Work out the finished part from the listing and answer in its coordinate system (mm). Round coordinates to 2 decimals unless told otherwise and drop trailing zeros. Write each loop counter-clockwise with the first axis right and the second up, starting at its lowest first coordinate (ties: lowest second). Pieces come first, ordered by that corner, then holes. Notation, with made-up numbers: M -4,-10.75 L 36,-10.75 A18 cw 36,-3.75 Z; hole C 29.25,73.5 d4. An arc over 180 degrees is marked long. Answer in a Markdown table with one row per item.
Autodesk Inventor part; units mm, degrees
ref_plane "YZ Plane" through (0, 0, 0) normal (1, 0, 0) x (0, 1, 0)
ref_plane "XZ Plane" through (0, 0, 0) normal (0, 1, 0) x (-1, 0, 0)
ref_plane "XY Plane" through (0, 0, 0) normal (0, 0, 1) x (1, 0, 0)
sketch "Sketch1" plane through (0, 0, 0) normal (0, 1, 0) x (-1, 0, 0)
  line L0 (0, 0) -> (48.3, 0)
  line L1 (48.3, 0) -> (48.3, -15)
  line L2 (48.3, -15) -> (0, -15)
  line L3 (0, -15) -> (0, 0)
  circle A0 centre (48.3, 0) radius 1.5
  circle A1 centre (48.3, -15) radius 1.5
  circle A2 centre (0, 0) radius 1.5
  circle A3 centre (0, -15) radius 1.5
  line L4 (48.3, -15) -> (52.3, -15)
  line L5 (52.3, -15) -> (52.3, -17.5)
  line L6 (52.3, -17.5) -> (48.3, -17.5)
  line L7 (48.3, -17.5) -> (48.3, -15)
  line L8 (0, 0) -> (-4, 0)
  line L9 (-4, 0) -> (-4, 2.5)
  line L10 (-4, 2.5) -> (0, 2.5)
  line L11 (0, 2.5) -> (0, 0)
  line L12 (-4, 2.5) -> (52.3, 2.5)
  line L13 (52.3, 2.5) -> (52.3, -17.5)
  line L14 (52.3, -17.5) -> (-4, -17.5)
  line L15 (-4, -17.5) -> (-4, 2.5)
  dimension "d0" = 48.3
  dimension "d1" = 15
  dimension "d2" = 3
  dimension "d3" = 3
  dimension "d4" = 3
  dimension "d5" = 3
  dimension "d6" = 4
  dimension "d7" = 2.5
  dimension "d8" = 4
  dimension "d9" = 2.5
extrude "Extrusion1" add sketch "Sketch1" along normal blind 2 contours A2 L11 L12 L13 L4 A1 L1 A0 L0 | L0 A0 L1 A1 L2 A3 L3 A2 | L3 A3 L2 A1 L7 L14 L15 L8 A2 | L8 L9 L10 L11 A2 | L7 A1 L4 L5 L6
sketch "Sketch2" plane through (0, 2, 0) normal (0, 1, 0) x (1, 0, 0)
  line L0 (4, -2.5) -> (4, 17.5)
  line L1 (4, -2.5) -> (-14.15, -2.5)
  line L2 (-14.15, -2.5) -> (-14.15, 7.5)
  line L3 (-14.15, 7.5) -> (4, 7.5)
  line L4 (4, 7.5) -> (4, -2.5)
  circle A0 centre (-14.15, 7.5) radius 3
  circle A1 centre (-14.15, 7.5) radius 1.5
  point P0 (0, 0)
  dimension "d12" = 18.15
  dimension "d13" = 10
  dimension "d14" = 6
  dimension "d19" = 3
extrude "Extrusion2" add sketch "Sketch2" along normal blind 1 contours A0 L2 A1 L3 | L3 A1 L2 A0
extrude "Extrusion3" cut sketch "Sketch2" against normal blind 3 contours A1 L2 L3 | L3 L2 A1
fillet "Fillet2" radius 2 1 edges at (-17.15, 2, -7.5)
properties part number "back_servo_support"
1. Determine the mould class of faces 1 (the flat face through (-24, 2, -7)), 2 (the cylindrical face through (-49.73, 0.99, -15.45)), 3 (the cylindrical face through (1.5, 0.99, -0.07)), 4 (the flat face through (-52.3, 1, -7)) for opening direction X: released by +X, released by -X, zero draft, split by the parting line, or undercut.
Calculated:
| item | result |
|---|---|
| face 1 | zero draft |
| face 2 | undercut |
| face 3 | undercut |
| face 4 | released by -X |
2. The part is cut by section A-A (x = 0). Determine the outline of the cut face in (y, z).
Calculated:
| item | result |
|---|---|
| outline | M 0,-17.5 L 2,-17.5 L 2,-16.5 L 0,-16.5 Z; M 0,-13.5 L 2,-13.5 L 2,-1.5 L 0,-1.5 Z; M 0,1.5 L 2,1.5 L 2,2.5 L 0,2.5 Z |
3. Consider line 1 along Z through (x, y) = (-48.3, 1); line 2 along X through (y, z) = (1.25, 0); line 3 along Z through (x, y) = (-47.5, 1.45). Determine where each line is inside the solid, lowest interval first. Write a range as from..to.
Calculated:
| item | result |
|---|---|
| line 1 | z = -17.5..-16.5, -13.5..-1.5, 1.5..2.5 |
| line 2 | x = -52.3..-49.8, -46.8..-1.5, 1.5..4 |
| line 3 | z = -17.5..-16.27, -13.73..-1.27, 1.27..2.5 |
4. The part is cut by section C-C (y = 1.5). Determine the outline of the cut face in (x, z), plus the area to 3 significant figures.
Calculated:
| item | result |
|---|---|
| outline | M -52.3,-17.5 L 4,-17.5 L 4,2.5 L -52.3,2.5 Z; hole C -48.3,-15 d3; hole C -48.3,0 d3; hole C -14.15,-7.5 d3; hole C 0,-15 d3; hole C 0,0 d3 |
| area | 1,090 mm² |
5. The part is cut by section B-B (z = -7.5). Determine the outline of the cut face in (x, y).
Calculated:
| item | result |
|---|---|
| outline | M -52.3,0 L -15.65,0 L -15.65,3 L -17.15,3 A2 cw -18.88,2 L -52.3,2 Z; M -12.65,0 L 4,0 L 4,2 L -9.42,2 A2 cw -11.15,3 L -12.65,3 Z |
6. The part is cut by section D-D (z = -15). Determine the outline of the cut face in (x, y).
Calculated:
| item | result |
|---|---|
| outline | M -52.3,0 L -49.8,0 L -49.8,2 L -52.3,2 Z; M -46.8,0 L -1.5,0 L -1.5,2 L -46.8,2 Z; M 1.5,0 L 4,0 L 4,2 L 1.5,2 Z |
